For this review, take the finished solid that the model builds, in its own axes (mm). Face numbers are marked on the shaded views. A direction names the side the tool comes from. Coordinates: 2 decimals unless noted, no trailing zeros. Order: outer loops, then holes, each group sorted by start corner. A loop starts at its lowest first (then second) coordinate and runs counter-clockwise, first axis right, second up. Notation, with made-up numbers: (40.5, 10.25) -> (59.5, 10.25) arc R34 cw to (59.5, 48.25) -> close; hole circle Ø8 at (-1.75, 64). An arc over 180 degrees is marked (long way). Return JSON: item names as keys, results as strings. Group by question number.
Item 1: Take a section at D-D (z = 8.75). Write out the cut boundary in (x, y).
Item 2: Take a section at B-B (z = 16.5). Write out the cut boundary in (x, y).
Item 3: Insertion check: pin 1 (0.7 mm diameter, centred on y = 12, z = 2, fed in from -X); pin 2 (3.5 mm diameter, centred on x = -8.5, z = 1, fed in from +Y); pin 3 (4 mm diameter, centred on x = 7.5, y = 7.5, fed in from +Z) (3 decimals). Each pin has a flat end and moves straight along its axis. Give the tip position at first contact, or say it passes through.
Item 4: Machinability: for the marked faces 1, 2 and 3, which of the approach directions +Z, -Z, +X, -X, +Y, -Y give a long, thin tool a straight path to every point of the face, cutting with its end or side? Answer none if there is none.
Item 5: Take a section at C-C (x = 7.5). Write out the cut boundary in (y, z) (3 decimals).
Item 6: Take a section at A-A (y = -4.25). Write out the cut boundary in (x, z) (3 decimals), then the cut area to 3 significant figures.
Item 7: For line 1 along Z through (x, y) = (9.75, 8.75) (3 decimals); line 2 along Y through (x, z) = (9.25, 4.5); line 3 along Z through (x, y) = (1, -5.25) (3 decimals), list the stretches that pass through material, from the lowest coordinate up.
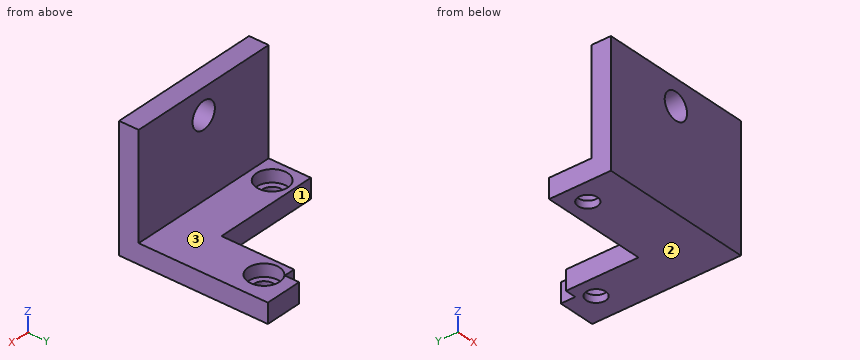
```python
from build123d import *

# Parameters (mm, degrees)
SKETCH2_R           = 1.5748
SKETCH2_W           = 1
SKETCH2_H           = 6.842
BOSS_EXTRUDE1_DEPTH = 3.175
SKETCH3_W           = 25.098
SKETCH3_H           = 3.175
BOSS_EXTRUDE3_DEPTH = 20
SKETCH4_R           = 2.159
CUT_EXTRUDE1_DEPTH  = 34.8656879
SKETCH5_R           = 2.54
CUT_EXTRUDE2_DEPTH  = 2


with BuildPart() as part:
    # Sketch2 → Boss-Extrude1 (new body)
    # profile 1 of 2: a face of its own
    with BuildSketch(Plane.XY):
        Polygon((4.395213829, 10.321811953), (4.395213829, 7.827388121), (4.395213829, -1.438404904), (-11.860786171, -1.438404904), (-11.860786171, -8.280404904), (12.237213829, -8.280404904), (12.237213829, 12.658595096), (7.697213829, 12.658595096), (6.188170382, 12.658595096), (6.188170382, 10.321811953), align=None)
        with Locations((-9.320786171, -4.740404904)):
            Circle(SKETCH2_R, mode=Mode.SUBTRACT)
        with Locations((7.697213829, 8.213595096)):
            Circle(SKETCH2_R, mode=Mode.SUBTRACT)
    # profile 2 of 2: a face of its own
    with BuildSketch(Plane.XY):
        with Locations((-12.360786171, -4.859404904)):
            Rectangle(SKETCH2_W, SKETCH2_H)
    extrude(amount=BOSS_EXTRUDE1_DEPTH)

    # Sketch3 → Boss-Extrude3 (add)
    with BuildSketch(Plane(origin=(0, 0, 0), x_dir=(-1, 0, 0), z_dir=(0, 0, -1))):
        with Locations((0.311786171, -9.867904904)):
            Rectangle(SKETCH3_W, SKETCH3_H)
    extrude(amount=-BOSS_EXTRUDE3_DEPTH)

    # Sketch4 → Cut-Extrude1 (cut, through all)
    with BuildSketch(Plane.XZ.offset(11.455404904)):
        with Locations(Location((-0.311786171, 15.875, 0), (0, 0, 270))):
            Circle(SKETCH4_R)
    extrude(amount=-CUT_EXTRUDE1_DEPTH, mode=Mode.SUBTRACT)

    # Sketch5 → Cut-Extrude2 (cut)
    with BuildSketch(Plane.XY.offset(3.175)):
        with Locations((7.697213829, 8.213595096)):
            Circle(SKETCH5_R)
        with Locations((-9.320786171, -4.740404904)):
            Circle(SKETCH5_R)
    extrude(amount=-CUT_EXTRUDE2_DEPTH, mode=Mode.SUBTRACT)


solid = part.part
```
Findings below:
{
 "1": {"outline": "(-12.86, -11.46) -> (12.24, -11.46) -> (12.24, -8.28) -> (-12.86, -8.28) -> close"},
 "2": {"outline": "(-12.86, -11.46) -> (-2.38, -11.46) -> (-2.38, -8.28) -> (-12.86, -8.28) -> close; (1.75, -11.46) -> (12.24, -11.46) -> (12.24, -8.28) -> (1.75, -8.28) -> close"},
 "3": {"pin 1": "stops at x = 6.19", "pin 2": "stops at y = -1.44", "pin 3": "stops at z = 3.175"},
 "4": {"face 1": "+Z, -Z, -X, +Y", "face 2": "-Z, +X, -X, +Y, -Y", "face 3": "+Z, +X, -X, +Y"},
 "5": {"outline": "(-11.455, 0) -> (6.651, 0) -> (6.651, 1.175) -> (5.681, 1.175) -> (5.681, 3.175) -> (-8.28, 3.175) -> (-8.28, 20) -> (-11.455, 20) -> close; (9.776, 0) -> (12.659, 0) -> (12.659, 3.175) -> (10.746, 3.175) -> (10.746, 1.175) -> (9.776, 1.175) -> close"},
 "6": {"outline": "(-12.861, 0) -> (-10.817, 0) -> (-10.817, 1.175) -> (-11.813, 1.175) -> (-11.813, 3.175) -> (-12.861, 3.175) -> close; (-7.824, 0) -> (12.237, 0) -> (12.237, 3.175) -> (-6.829, 3.175) -> (-6.829, 1.175) -> (-7.824, 1.175) -> close", "area": "66.2 mm2"},
 "7": {"line 1": "z = 0 to 1.175", "line 2": "y = -11.46 to -8.28", "line 3": "z = 0 to 3.175"}
}
